```python
from build123d import *

# Parameters (mm, degrees)
BOSS_EXTRUDE1_DEPTH      = 2.54
CUT_EXTRUDE1_DEPTH       = 2.54
CUT_EXTRUDE3_START       = -2.54
SKETCH4_W                = 57.139047114
SKETCH4_H                = 47.329047114
CUT_EXTRUDE3_DEPTH       = 2.54
FILLET5_R                = 1.27
FILLET6_R                = 1.27
FILLET7_R                = 2.54
BOSS_EXTRUDE2_DEPTH      = 10.16
BOSS_EXTRUDE2_DEPTH_BACK = 10.16
SKETCH7_W                = 15.24
SKETCH7_H                = 106.095476443
CUT_EXTRUDE4_DEPTH       = 52.324
SKETCH8_W                = 15.24
SKETCH8_H                = 12.7
SKETCH8_R                = 1.524
BOSS_EXTRUDE3_DEPTH      = 2.54
SKETCH10_W               = 14.001226512
SKETCH10_H               = 1.640904711
CUT_EXTRUDE5_DEPTH       = 12.192
FILLET9_R                = 1.27
FILLET10_R               = 1.27
SKETCH11_W               = 15.296857303
SKETCH11_H               = 2.54
BOSS_EXTRUDE4_DEPTH      = 2.54
FILLET12_R               = 1.27


with BuildPart() as part:
    # Sketch1 → Boss-Extrude1 (new body)
    with BuildSketch(Plane(origin=(0, 0, 0), x_dir=(-1, 0, 0), z_dir=(0, 0, 1))):
        with BuildLine():
            Line((-27.900000003, -31.869047114), (27.899999998, -31.869047114))
            ThreePointArc((27.899999998, -31.869047114), (30.70654013, -30.706540129), (31.869047114, -27.899999998))
            Line((31.869047114, -27.899999998), (31.869047114, 27.899999996))
            ThreePointArc((31.869047114, 27.899999996), (30.70654013, 30.706540129), (27.899999998, 31.869047114))
            Line((27.899999998, 31.869047114), (-27.899999996, 31.869047114))
            ThreePointArc((-27.899999996, 31.869047114), (-30.706540129, 30.70654013), (-31.869047114, 27.899999998))
            Line((-31.869047114, 27.899999998), (-31.869047114, -27.900000002))
            ThreePointArc((-31.869047114, -27.900000002), (-30.70654013, -30.706540129), (-27.900000003, -31.869047114))
        make_face()
        with BuildLine():
            ThreePointArc((-25.5, 18), (-24, 16.5), (-22.5, 18))
            ThreePointArc((-22.5, 18), (-24, 19.5), (-25.5, 18))
        make_face(mode=Mode.SUBTRACT)
        with BuildLine():
            ThreePointArc((22.5, 18), (24, 16.5), (25.5, 18))
            ThreePointArc((25.5, 18), (24, 19.5), (22.5, 18))
        make_face(mode=Mode.SUBTRACT)
        with BuildLine():
            ThreePointArc((25.5, -18), (24, -16.5), (22.5, -18))
            ThreePointArc((22.5, -18), (24, -19.5), (25.5, -18))
        make_face(mode=Mode.SUBTRACT)
        with BuildLine():
            ThreePointArc((-22.5, -18), (-24, -16.5), (-25.5, -18))
            ThreePointArc((-25.5, -18), (-24, -19.5), (-22.5, -18))
        make_face(mode=Mode.SUBTRACT)
    extrude(amount=BOSS_EXTRUDE1_DEPTH)

    # Sketch2 → Cut-Extrude1 (cut)
    with BuildSketch(Plane.XY.offset(2.54)):
        Polygon((-16.38, 15.46), (0, 3.175), (16.38, 15.46), align=None)
        Polygon((21.46, 12.92), (21.46, -12.92), (4.233333333, 0), align=None)
        Polygon((-21.46, -12.92), (-21.46, 12.92), (-4.233333333, 0), align=None)
        Polygon((0, -3.175), (16.38, -15.46), (-16.38, -15.46), align=None)
    extrude(amount=-CUT_EXTRUDE1_DEPTH, mode=Mode.SUBTRACT)

    # Sketch4 → Cut-Extrude3 (cut)
    with BuildSketch(Plane.XY.offset(2.54).offset(CUT_EXTRUDE3_START)):
        with BuildLine():
            Line((27.900000003, 31.869047114), (-27.899999998, 31.869047114))
            ThreePointArc((-27.899999998, 31.869047114), (-30.70654013, 30.706540129), (-31.869047114, 27.899999998))
            Line((-31.869047114, 27.899999998), (-31.869047114, -27.899999996))
            ThreePointArc((-31.869047114, -27.899999996), (-30.70654013, -30.706540129), (-27.899999998, -31.869047114))
            Line((-27.899999998, -31.869047114), (27.899999996, -31.869047114))
            ThreePointArc((27.899999996, -31.869047114), (30.706540129, -30.70654013), (31.869047114, -27.899999998))
            Line((31.869047114, -27.899999998), (31.869047114, 27.900000002))
            ThreePointArc((31.869047114, 27.900000002), (30.70654013, 30.706540129), (27.900000003, 31.869047114))
        make_face()
        Rectangle(SKETCH4_W, SKETCH4_H, mode=Mode.SUBTRACT)
    extrude(amount=CUT_EXTRUDE3_DEPTH, mode=Mode.SUBTRACT)

    # Fillet5
    fillet5_edges = [part.edges().sort_by_distance(p)[0] for p in [
        (16.38, 15.46, 1.27),
        (-16.38, 15.46, 1.27),
        (-21.46, 12.92, 1.27),
        (-21.46, -12.92, 1.27),
        (16.38, -15.46, 1.27),
        (-16.38, -15.46, 1.27),
        (21.46, 12.92, 1.27),
        (21.46, -12.92, 1.27),
    ]]
    fillet(fillet5_edges, radius=FILLET5_R)

    # Fillet6
    fillet6_edges = [part.edges().sort_by_distance(p)[0] for p in [
        (0, 3.175, 1.27),
        (-4.233333333, 0, 1.27),
        (0, -3.175, 1.27),
        (4.233333333, 0, 1.27),
    ]]
    fillet(fillet6_edges, radius=FILLET6_R)

    # Fillet7
    fillet7_edges = [part.edges().sort_by_distance(p)[0] for p in [
        (28.569523557, -23.664523557, 1.27),
        (-28.569523557, -23.664523557, 1.27),
        (-28.569523557, 23.664523557, 1.27),
        (28.569523557, 23.664523557, 1.27),
    ]]
    fillet(fillet7_edges, radius=FILLET7_R)

    # Sketch6 → Boss-Extrude2 (add, two sides: drawn at the far end of the back side and taken through both)
    with BuildSketch(Plane(origin=(0, 0, 0), x_dir=(0, 0, -1), z_dir=(1, 0, 0)).offset(-BOSS_EXTRUDE2_DEPTH_BACK)):
        Polygon((-2.54, -129.76), (-2.54, -23.664523557), (-2.54, -15.46), (0, -15.46), (22.86, -129.76), align=None)
    extrude(amount=BOSS_EXTRUDE2_DEPTH + BOSS_EXTRUDE2_DEPTH_BACK)

    # Sketch7 → Cut-Extrude4 (cut)
    with BuildSketch(Plane.XY.offset(2.54)):
        with Locations((0, -76.712261779)):
            Rectangle(SKETCH7_W, SKETCH7_H)
    extrude(amount=-CUT_EXTRUDE4_DEPTH, mode=Mode.SUBTRACT)

    # Sketch8 → Boss-Extrude3 (add)
    with BuildSketch(Plane.XZ.offset(129.76)):
        Polygon((-15.24, 2.54), (-15.24, -3.81), (-10.16, -3.81), (-10.16, -22.86), (10.16, -22.86), (10.16, -3.81), (15.24, -3.81), (15.24, 2.54), align=None)
        with Locations((0, -10.16)):
            Rectangle(SKETCH8_W, SKETCH8_H, mode=Mode.SUBTRACT)
        with Locations(Location((-12.7, -0.635, 0), (0, 0, 270))):
            Circle(SKETCH8_R, mode=Mode.SUBTRACT)
        with Locations(Location((12.7, -0.635, 0), (0, 0, 270))):
            Circle(SKETCH8_R, mode=Mode.SUBTRACT)
        with Locations(Location((0, -19.685, 0), (0, 0, 270))):
            Circle(SKETCH8_R, mode=Mode.SUBTRACT)
    extrude(amount=BOSS_EXTRUDE3_DEPTH)

    # Sketch10 → Cut-Extrude5 (cut)
    with BuildSketch(Plane.XZ.offset(23.664523557)):
        with Locations((0.619386744, -0.820452356)):
            Rectangle(SKETCH10_W, SKETCH10_H)
    extrude(amount=-CUT_EXTRUDE5_DEPTH, mode=Mode.SUBTRACT)

    # Fillet9
    fillet9_edges = [part.edges().sort_by_distance(p)[0] for p in [
        (7.62, -23.664523557, 1.27),
        (-7.62, -23.664523557, 0.449547644),
        (-10.16, -23.664523557, 1.27),
        (10.16, -23.664523557, 1.27),
    ]]
    fillet(fillet9_edges, radius=FILLET9_R)

    # Fillet10
    fillet10_edges = [part.edges().sort_by_distance(p)[0] for p in [
        (7.62, -131.03, -3.81),
        (7.62, -131.03, -16.51),
        (-7.62, -131.03, -16.51),
        (10.16, -131.03, -3.81),
        (15.24, -131.03, -3.81),
        (15.24, -131.03, 2.54),
        (-15.24, -131.03, 2.54),
        (-15.24, -131.03, -3.81),
        (-7.62, -131.03, -3.81),
        (-10.16, -131.03, -3.81),
    ]]
    fillet(fillet10_edges, radius=FILLET10_R)

    # Sketch11 → Boss-Extrude4 (add)
    with BuildSketch(Plane.XY.offset(2.54)):
        with Locations((-0.028428652, -76.712261779)):
            Rectangle(SKETCH11_W, SKETCH11_H)
    extrude(amount=-BOSS_EXTRUDE4_DEPTH)

    # Fillet12
    fillet12_edges = [part.edges().sort_by_distance(p)[0] for p in [
        (-7.62, -75.442261779, 1.27),
        (-7.62, -77.982261779, 1.27),
        (7.62, -77.982261779, 1.27),
        (7.62, -75.442261779, 1.27),
    ]]
    fillet(fillet12_edges, radius=FILLET12_R)


solid = part.part
```
Work out the finished part from the listing and answer in its coordinate system (mm). A direction names the side the tool comes from. Coordinates: 2 decimals unless noted, no trailing zeros. Write each loop counter-clockwise with the first axis right and the second up, starting at its lowest first coordinate (ties: lowest second). Pieces come first, ordered by that corner, then holes.
Q1. Determine the mould class of faces 6 (the face through (0, -23.665, 1)), 7 (the face through (-2, -19, 2.54)), 8 (the face through (27.806, 22.94, 1.288)), 9 (the face through (0, -75.442, 1)) for opening direction Y: released by +Y, released by -Y, zero draft, split by the parting line, or undercut.
Q2. A cutting plane is placed at A-A, the plane z = -12. Give the vertices of the cut face in (x, y), then the cut area to 3 significant figures.
Q3. Each of these flat-tipped pins is pushed along its axis until it touches: pin 1 Ø2.5 at (x, z) = (3, -2.5) entering from +Y; pin 2 Ø2 at (y, z) = (-131, -1) entering from +X; pin 3 Ø2 at (x, y) = (-9, -17.5) entering from -Z. Where does it stop, or does it pass through?
Q4. A cutting plane is placed at C-C, the plane y = -18. Give the vertices of the cut face in (x, z), then the cut area to 3 significant figures.
Q5. A cutting plane is placed at B-B, the plane x = 24. Give the vertices of the cut face in (y, z).
Q6. Which of the six approach directions +Z, -Z, +X, -X, +Y, -Y give full straight-line access (tool end or side, diameter ignored) to faces 1 (the face through (15.24, -131, -1)), 2 (the face through (-8.72, -71.81, -11.27)), 3 (the face through (19, -23.665, 1)), 4 (the face through (0, -131, -16.51)), 5 (the face through (-12.605, 6.279, 1.288))?
Q7. A cutting plane is placed at D-D, the plane x = -18. Give the vertices of the cut face in (y, z) (3 decimals).
Q8. Find the intervals of material crossed by line 1 (Y direction, x = 24, z = 1.2); line 2 (X direction, y = -50, z = -4); line 3 (X direction, y = -18, z = 1.8), in increasing order.
Findings below:
1. face 6: undercut
1. face 7: zero draft
1. face 8: released by +Y
1. face 9: undercut
2. outline: (-10.16, -132.3) - (-7.62, -132.3) - (-7.62, -75.46) - (-10.16, -75.46) - close; (7.62, -132.3) - (10.16, -132.3) - (10.16, -75.46) - (7.62, -75.46) - close
2. area: 289 mm2
3. pin 1: stops at y = -129.76
3. pin 2: stops at x = 15.24
3. pin 3: stops at z = -0.61
4. outline: (-28.57, 0) - (-25.5, 0) - (-25.5, 2.54) - (-28.57, 2.54) - close; (-22.5, 0) - (-10.16, 0) - (-10.16, -0.51) - (-6.38, -0.51) - (-6.38, 0) - (7.62, 0) - (7.62, -0.51) - (10.16, -0.51) - (10.16, 0) - (22.5, 0) - (22.5, 2.54) - (-22.5, 2.54) - close; (25.5, 0) - (28.57, 0) - (28.57, 2.54) - (25.5, 2.54) - close
4. area: 133 mm2
5. outline: (-23.66, 0) - (-19.5, 0) - (-19.5, 2.54) - (-23.66, 2.54) - close; (-16.5, 0) - (16.5, 0) - (16.5, 2.54) - (-16.5, 2.54) - close; (19.5, 0) - (23.66, 0) - (23.66, 2.54) - (19.5, 2.54) - close
6. face 1: +Z, -Z, +X, -Y
6. face 2: -Z, +X, -X, +Y
6. face 3: +Z, -Z, +X
6. face 4: +Y, -Y
6. face 5: +Z, -Z
7. outline: (-23.665, 0) - (-10.325, 0) - (-10.325, 2.54) - (-23.665, 2.54) - close; (10.325, 0) - (23.665, 0) - (23.665, 2.54) - (10.325, 2.54) - close
8. line 1: y = -23.66 to -19.5, -16.5 to 16.5, 19.5 to 23.66
8. line 2: x = -10.16 to -7.62, 7.62 to 10.16
8. line 3: x = -28.57 to -25.5, -22.5 to 22.5, 25.5 to 28.57
